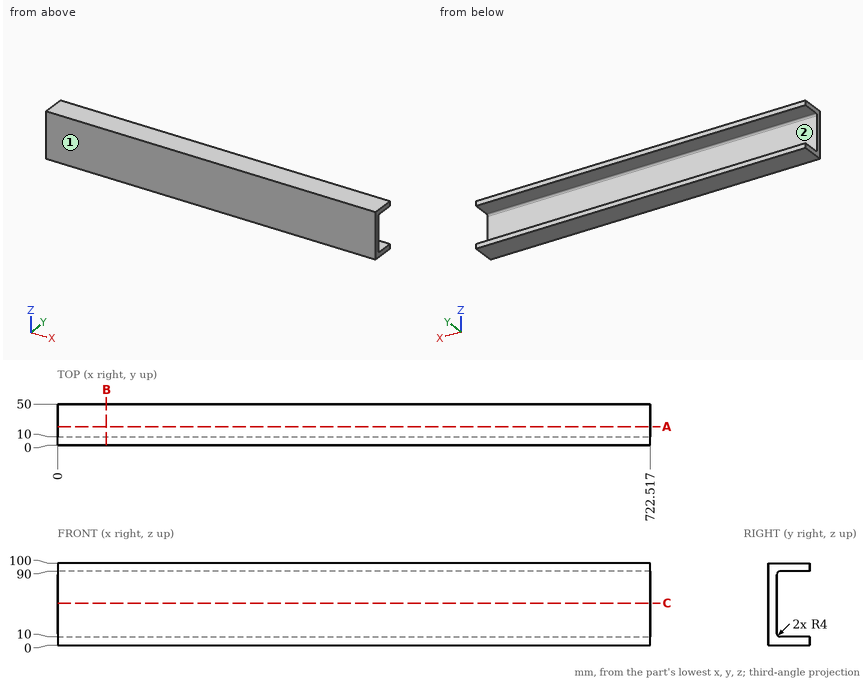
Can you work these out from the drawing? Everything is in mm from the part's minimum corner. Round coordinates to 2 decimals unless told otherwise and drop trailing zeros. Loops run counter-clockwise (first coordinate to the right, second up) from the corner with the lowest first, then second, coordinate; pieces in that order, holes last. Notation, with made-up numbers: (-4.75, 32.25) - (27.25, 32.25) arc R24 ccw to (27.25, 49.25) - close; hole circle Ø2 at (42, 12.5). An arc over 180 degrees is marked (long way). Answer as CSV lines item,"result".
1. For pin 1 Ø12 at (y, z) = (31, 79) entering from -X; pin 2 Ø1.5 at (x, z) = (643.5, 69.5) entering from +Y, each with a flat end and sliding along its axis, tell me the tip position at first contact or that it passes through.
Filled in:
pin 1,"passes through"
pin 2,"stops at y = 10"
2. I want a section at C-C on z = 51. List the corners of the cut face in (x, y) for me.
Filled in:
outline,"(0, 0) - (722.52, 0) - (722.52, 10) - (0, 10) - close"
3. We'd pull the mould along Z, two halves only. Please class the marked faces 1 and 2: +Z half, -Z half, draft (parallel to the pull), parting line (faces both ways), or undercut.
Filled in:
face 1,"draft"
face 2,"undercut"
4. Please list where these lines run through material, in increasing order: line 1 along Z through (x, y) = (245, 20); line 2 along Y through (x, z) = (505.5, 84.5); line 3 along Z through (x, y) = (318.5, 12.5). Write a range as [from, to].
Filled in:
line 1,"z = [0, 10], [90, 100]"
line 2,"y = [0, 10]"
line 3,"z = [0, 10.29], [89.71, 100]"
5. I want a section at A-A on y = 22.5. List the corners of the cut face in (x, z) for me.
Filled in:
outline,"(0, 0) - (722.52, 0) - (722.52, 10) - (0, 10) - close; (0, 90) - (722.52, 90) - (722.52, 100) - (0, 100) - close"
6. I want a section at B-B on x = 59.5. List the corners of the cut face in (y, z) for me, then the cut area to 3 significant figures.
Filled in:
outline,"(0, 0) - (50, 0) - (50, 10) - (14, 10) arc R4 cw to (10, 14) - (10, 86) arc R4 cw to (14, 90) - (50, 90) - (50, 100) - (0, 100) - close"
area,"1,810 mm^2"
